Geometry check sheet. Reference: the model listing, model coordinates, mm. Give positions to 0.01 mm unless a question says otherwise; leave off trailing zeros. Loops run counter-clockwise (first coordinate to the right, second up) from the corner with the lowest first, then second, coordinate; pieces in that order, holes last. Notation, with made-up numbers: (80.25, 84) -> (114.25, 84) arc R14 ccw to (114.25, 91) -> close; hole circle Ø10 at (19.5, -11). An arc over 180 degrees is marked (long way). Write each question's results on one line, items separated by ' | '. Start each with the question number.
1) Sectioned sample at B-B on z = 40. Record the cut outline in (x, y).
2) Sectioned sample at D-D on x = 137. Record the cut outline in (y, z).
3) Depth check by flat-ended pin: pin 1 (24 mm diameter, centred on x = -137, z = 40, fed in from +Y). Enter the tip coordinate at first touch or a pass-through.
4) Sectioned sample at C-C on y = 1.1. Record the cut outline in (x, z), then the cut area to 3 significant figures.
5) Scan lines: line 1 (X direction, y = 1, z = 40); line 2 (Z direction, x = 132.5, y = 2.25); line 3 (X direction, y = 1.1, z = -49). Record each from-to range of solid material in increasing order. Write a range as from..to.
6) Sectioned sample at A-A on x = 0. Record the cut outline in (y, z), then the cut area to 3 significant figures.
```python
from build123d import *

# Parameters (mm, degrees)
SKETCH1_W           = 314
SKETCH1_H           = 120
SKETCH1_R           = 24.5
SKETCH1_R_2         = 10.5
BOSS_EXTRUDE1_DEPTH = 3
FILLET1_R           = 3


with BuildPart() as part:
    # Sketch1 → Boss-Extrude1 (new body)
    with BuildSketch(Plane(origin=(0, 0, 0), x_dir=(1, 0, 0), z_dir=(0, 1, 0))):
        Rectangle(SKETCH1_W, SKETCH1_H)
        with Locations(Location((0, 0, 0), (0, 0, 270))):
            Circle(SKETCH1_R, mode=Mode.SUBTRACT)
        with Locations(Location((-137, 40, 0), (0, 0, 270))):
            Circle(SKETCH1_R_2, mode=Mode.SUBTRACT)
        with Locations(Location((137, 40, 0), (0, 0, 90))):
            Circle(SKETCH1_R_2, mode=Mode.SUBTRACT)
        with Locations(Location((137, -40, 0), (0, 0, 270))):
            Circle(SKETCH1_R_2, mode=Mode.SUBTRACT)
        with Locations(Location((-137, -40, 0), (0, 0, 90))):
            Circle(SKETCH1_R_2, mode=Mode.SUBTRACT)
    extrude(amount=BOSS_EXTRUDE1_DEPTH)

    # Fillet1
    fillet1_edges = [part.edges().sort_by_distance(p)[0] for p in [
        (157, 1.5, -60),
        (157, 1.5, 60),
        (-157, 1.5, 60),
        (-157, 1.5, -60),
    ]]
    fillet(fillet1_edges, radius=FILLET1_R)


solid = part.part
```
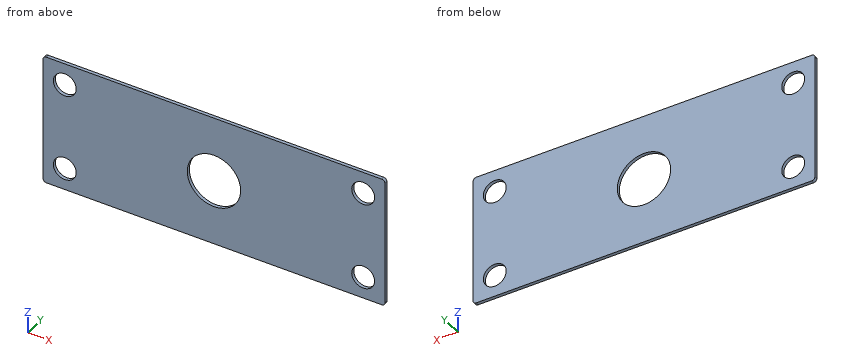
Result:
1) outline: (-157, 0) -> (-147.5, 0) -> (-147.5, 3) -> (-157, 3) -> close; (-126.5, 0) -> (126.5, 0) -> (126.5, 3) -> (-126.5, 3) -> close; (147.5, 0) -> (157, 0) -> (157, 3) -> (147.5, 3) -> close
2) outline: (0, -60) -> (3, -60) -> (3, -50.5) -> (0, -50.5) -> close; (0, -29.5) -> (3, -29.5) -> (3, 29.5) -> (0, 29.5) -> close; (0, 50.5) -> (3, 50.5) -> (3, 60) -> (0, 60) -> close
3) pin 1: y = 3
4) outline: (-157, -57) arc R3 ccw to (-154, -60) -> (154, -60) arc R3 ccw to (157, -57) -> (157, 57) arc R3 ccw to (154, 60) -> (-154, 60) arc R3 ccw to (-157, 57) -> close; hole circle Ø21 at (-137, -40); hole circle Ø21 at (-137, 40); hole circle Ø49 at (0, 0); hole circle Ø21 at (137, -40); hole circle Ø21 at (137, 40) | area: 34,400 mm^2
5) line 1: -157..-147.5, -126.5..126.5, 147.5..157 | line 2: -60..-49.49, -30.51..30.51, 49.49..60 | line 3: -157..-142.41, -131.59..131.59, 142.41..157
6) outline: (0, -60) -> (3, -60) -> (3, -24.5) -> (0, -24.5) -> close; (0, 24.5) -> (3, 24.5) -> (3, 60) -> (0, 60) -> close | area: 213 mm^2
